Read the model definition and answer for the solid it produces. Units are mm, in the model's axes. A direction names the side the tool comes from. Coordinates: 2 decimals unless noted, no trailing zeros. Write each loop counter-clockwise with the first axis right and the second up, starting at its lowest first coordinate (ties: lowest second). Pieces come first, ordered by that corner, then holes. Notation, with made-up numbers: (31, 66.25) - (83, 66.25) arc R11 cw to (83, 77.25) - close; hole circle Ø1 at (1, 45). An arc over 180 degrees is marked (long way). Use a Markdown table: item, result.
from build123d import *

# Parameters (mm, degrees)
PAD_DEPTH    = 30
PAD001_DEPTH = 10
PAD002_DEPTH = 10


with BuildPart() as part:
    # Sketch → Pad (new body)
    with BuildSketch(Plane.XY):
        Polygon((-4.997332, 9), (-2.497332, 9), (-2.497332, 8), (-2.997332, 8), (-2.997332, 4), (37.102668, 4), (37.102668, 8), (36.602668, 8), (36.602668, 9), (39.102668, 9), (39.102668, 0), (-4.997332, 0), (-4.997332, 4), align=None)
    extrude(amount=PAD_DEPTH)

    # Sketch001 (on Face10 of Pad) → Pad001 (join)
    with BuildSketch(Plane.YZ.offset(9.602668)):
        Polygon((0.1, 0), (0.1, 3), (-90.4, 3), (-90.4, 11.5), (-88.552241, 12.265367), (-90.4, 13.030734), (-93.4, 13.030734), (-93.4, 0), align=None)
    extrude(amount=PAD001_DEPTH)

    # Sketch002 (on Face10 of Pad) → Pad002 (join)
    with BuildSketch(Plane.YZ.offset(27.202668)):
        Polygon((0.1, 0), (0.1, 3), (-90.4, 3), (-90.4, 11.5), (-88.552241, 12.265367), (-90.4, 13.030734), (-93.4, 13.030734), (-93.4, 0), align=None)
    extrude(amount=PAD002_DEPTH)


solid = part.part
(1) A cutting plane is placed at B-B, the plane y = -19.5. Write down the section's boundary in (x, z), and give its area (3 significant figures).
Report:
| item | result |
|---|---|
| outline | (9.6, 0) - (19.6, 0) - (19.6, 3) - (9.6, 3) - close; (27.2, 0) - (37.2, 0) - (37.2, 3) - (27.2, 3) - close |
| area | 60.0 mm² |
(2) A cutting plane is placed at D-D, the plane z = 19. Write down the section's boundary in (x, y), and give its area (3 significant figures).
Report:
| item | result |
|---|---|
| outline | (-5, 0) - (39.1, 0) - (39.1, 9) - (36.6, 9) - (36.6, 8) - (37.1, 8) - (37.1, 4) - (-3, 4) - (-3, 8) - (-2.5, 8) - (-2.5, 9) - (-5, 9) - close |
| area | 197 mm² |
(3) The mould has two halves that part along X. Classify faces 1 (the flat face through (37.103, 6, 15)), 2 (the flat face through (38, 9, 15)), 3 (the flat face through (-4.997, 5, 15)), 4 (the flat face through (37.203, -53.8, 2.7)): pulls with the +X half, pulls with the -X half, needs draft (parallel to the pull), parting line crosses it, or undercut.
Report:
| item | result |
|---|---|
| face 1 | undercut |
| face 2 | needs draft |
| face 3 | pulls with the -X half |
| face 4 | pulls with the +X half |
(4) Each of these flat-tipped pins is pushed along its axis until it touches: P1, Ø12, axis at x = 16, y = -53.5, coming from the +Z side; P2, Ø10.5, axis at y = -69.5, z = 4, coming from the +X side; P3, Ø4, axis at x = 15, z = 7.5, coming from the +Y side. Where does it stop, or does it pass through?
Report:
| item | result |
|---|---|
| P1 | stops at z = 3 |
| P2 | stops at x = 37.2 |
| P3 | stops at y = 4 |
(5) A cutting plane is placed at A-A, the plane z = 5.25. Write down the section's boundary in (x, y), and give its area (3 significant figures).
Report:
| item | result |
|---|---|
| outline | (-5, 0) - (39.1, 0) - (39.1, 9) - (36.6, 9) - (36.6, 8) - (37.1, 8) - (37.1, 4) - (-3, 4) - (-3, 8) - (-2.5, 8) - (-2.5, 9) - (-5, 9) - close; (9.6, -93.4) - (19.6, -93.4) - (19.6, -90.4) - (9.6, -90.4) - close; (27.2, -93.4) - (37.2, -93.4) - (37.2, -90.4) - (27.2, -90.4) - close |
| area | 257 mm² |
(6) A cutting plane is placed at C-C, the plane x = 14. Write down the section's boundary in (y, z), and give its area (3 significant figures).
Report:
| item | result |
|---|---|
| outline | (-93.4, 0) - (4, 0) - (4, 30) - (0, 30) - (0, 3) - (-90.4, 3) - (-90.4, 11.5) - (-88.55, 12.27) - (-90.4, 13.03) - (-93.4, 13.03) - close |
| area | 432 mm² |
(7) For faces 5 (the flat face through (17, -41, 0)), 6 (the flat face through (19.603, -53.8, 2.7)), 7 (the flat face through (14.533, -89.489, 11.877)), 8 (the flat face through (32.13, -89.46, 12.64)), 9 (the flat face through (9.603, -53.8, 2.7)), determine the directions among +Z, -Z, +X, -X, +Y, -Y from which every point of the face is accessible in a straight line to the end or side of a thin tool.
Report:
| item | result |
|---|---|
| face 5 | -Z, +X, -X, +Y, -Y |
| face 6 | +Z, -Z, -Y |
| face 7 | +X, -X |
| face 8 | +Z, +X, -X |
| face 9 | +Z, -Z, -X, -Y |
(8) Straight lines are drawn through the part: L1, parallel to Y at x = 29, z = 8.75; L2, parallel to X at y = -48, z = 2.25; L3, parallel to Y at x = 12.5, z = 19.25. For each, find the intervals that lie inside material, in ascending order.
Report:
| item | result |
|---|---|
| L1 | y = -93.4 to -90.4, 0 to 4 |
| L2 | x = 9.6 to 19.6, 27.2 to 37.2 |
| L3 | y = 0 to 4 |
